```python
from build123d import *

# Parameters (mm, degrees)
MODEL_R             = 3.175
BOSS_EXTRUDE1_DEPTH = 3.048
SKETCH2_R           = 1.4224
BOSS_EXTRUDE2_DEPTH = 3.048
SKETCH3_R           = 1.4224
SKETCH3_R_2         = 0.475
CUT_EXTRUDE1_DEPTH  = 47.828124767


with BuildPart() as part:
    # Model → Boss-Extrude1 (new body)
    with BuildSketch(Plane.XY):
        with BuildLine():
            ThreePointArc((-0.616026415, 14.286925194), (-1.042592722, 15.739677645), (-1.800954663, 17.050149187))
            ThreePointArc((-1.800954663, 17.050149187), (-2.148838289, 17.009806554), (-2.495825317, 16.962366609))
            ThreePointArc((-2.495825317, 16.962366609), (-2.904460903, 15.504468994), (-2.956341002, 13.991274707))
            ThreePointArc((-2.956341002, 13.991274707), (-3.556315124, 13.850932921), (-4.149686627, 13.684875627))
            ThreePointArc((-4.149686627, 13.684875627), (-4.924136412, 14.985904462), (-5.984574038, 16.066608185))
            ThreePointArc((-5.984574038, 16.066608185), (-6.311495456, 15.941017851), (-6.635783413, 15.808776154))
            ThreePointArc((-6.635783413, 15.808776154), (-6.669016568, 14.295057536), (-6.342950641, 12.816500973))
            ThreePointArc((-6.342950641, 12.816500973), (-6.88917389, 12.531360786), (-7.422606766, 12.222954996))
            ThreePointArc((-7.422606766, 12.222954996), (-8.496278501, 13.290511787), (-9.792160616, 14.073543103))
            ThreePointArc((-9.792160616, 14.073543103), (-10.077578151, 13.870596369), (-10.358790833, 13.661862153))
            ThreePointArc((-10.358790833, 13.661862153), (-10.014533394, 12.187435039), (-9.331009364, 10.836419348))
            ThreePointArc((-9.331009364, 10.836419348), (-9.789160524, 10.424397166), (-10.229137224, 9.993021149))
            ThreePointArc((-10.229137224, 9.993021149), (-11.534568165, 10.760027378), (-12.98446973, 11.196185548))
            ThreePointArc((-12.98446973, 11.196185548), (-13.210449547, 10.928634304), (-13.430917328, 10.656523107))
            ThreePointArc((-13.430917328, 10.656523107), (-12.730800257, 9.314031176), (-11.732766451, 8.175445642))
            ThreePointArc((-11.732766451, 8.175445642), (-12.0740582, 7.662430334), (-12.39293337, 7.135189032))
            ThreePointArc((-12.39293337, 7.135189032), (-13.84809849, 7.553450876), (-15.360916858, 7.615330478))
            ThreePointArc((-15.360916858, 7.615330478), (-15.513259815, 7.299985954), (-15.659129891, 6.981595523))
            ThreePointArc((-15.659129891, 6.981595523), (-14.647144119, 5.85539248), (-13.397310672, 5.000778618))
            ThreePointArc((-13.397310672, 5.000778618), (-13.600298394, 4.419004823), (-13.778035935, 3.829026746))
            ThreePointArc((-13.778035935, 3.829026746), (-15.291501858, 3.872263276), (-16.772181085, 3.555976188))
            ThreePointArc((-16.772181085, 3.555976188), (-16.841314914, 3.212652639), (-16.903421733, 2.867988616))
            ThreePointArc((-16.903421733, 2.867988616), (-15.643154047, 2.02883794), (-14.220052592, 1.511894283))
            ThreePointArc((-14.220052592, 1.511894283), (-14.271981822, 0.897916987), (-14.297413829, 0.282272628))
            ThreePointArc((-14.297413829, 0.282272628), (-15.774083925, -0.052232867), (-17.129587491, -0.726813165))
            ThreePointArc((-17.129587491, -0.726813165), (-17.111168259, -1.076543457), (-17.085609422, -1.425824564))
            ThreePointArc((-17.085609422, -1.425824564), (-15.656247076, -1.92519595), (-14.14929631, -2.071987931))
            ThreePointArc((-14.14929631, -2.071987931), (-14.046904143, -2.679590275), (-13.918432631, -3.282217718))
            ThreePointArc((-13.918432631, -3.282217718), (-15.265522286, -3.973447027), (-16.410678917, -4.963934173))
            ThreePointArc((-16.410678917, -4.963934173), (-16.305863972, -5.298096369), (-16.194245434, -5.630047943))
            ThreePointArc((-16.194245434, -5.630047943), (-14.68560052, -5.758262697), (-13.189487703, -5.525679522))
            ThreePointArc((-13.189487703, -5.525679522), (-12.939207816, -6.088729025), (-12.664905121, -6.640474253))
            ThreePointArc((-12.664905121, -6.640474253), (-13.797771739, -7.644994897), (-14.660627033, -8.889152941))
            ThreePointArc((-14.660627033, -8.889152941), (-14.476002283, -9.1867504), (-14.285337446, -9.480514703))
            ThreePointArc((-14.285337446, -9.480514703), (-12.792203675, -9.229516622), (-11.400935076, -8.632172348))
            ThreePointArc((-11.400935076, -8.632172348), (-11.018493474, -9.115290538), (-10.615595045, -9.581485369))
            ThreePointArc((-10.615595045, -9.581485369), (-11.46305645, -10.836179621), (-11.989394033, -12.255833538))
            ThreePointArc((-11.989394033, -12.255833538), (-11.736560131, -12.498167117), (-11.47882917, -12.735285858))
            ThreePointArc((-11.47882917, -12.735285858), (-10.095025626, -12.120846074), (-8.896019768, -11.196274037))
            ThreePointArc((-8.896019768, -11.196274037), (-8.405446665, -11.569104823), (-7.899268091, -11.920456521))
            ThreePointArc((-7.899268091, -11.920456521), (-8.408075165, -13.346487327), (-8.564823313, -14.85243504))
            ThreePointArc((-8.564823313, -14.85243504), (-8.259666742, -15.024278029), (-7.95106384, -15.189852165))
            ThreePointArc((-7.95106384, -15.189852165), (-6.76353999, -14.25057819), (-5.832134822, -13.056872652))
            ThreePointArc((-5.832134822, -13.056872652), (-5.264254728, -13.295989703), (-4.686601071, -13.510421549))
            ThreePointArc((-4.686601071, -13.510421549), (-4.824783595, -15.018186149), (-4.602093245, -16.515803425))
            ThreePointArc((-4.602093245, -16.515803425), (-4.263788115, -16.606358298), (-3.923703928, -16.689984197))
            ThreePointArc((-3.923703928, -16.689984197), (-3.007076261, -15.484894068), (-2.401795395, -14.097059939))
            ThreePointArc((-2.401795395, -14.097059939), (-1.792290307, -14.187438652), (-1.17945767, -14.251477104))
            ThreePointArc((-1.17945767, -14.251477104), (-0.938333127, -15.746237102), (-0.350196733, -17.14142314))
            ThreePointArc((-0.350196733, -17.14142314), (0, -17.145), (0.350196733, -17.14142314))
            ThreePointArc((0.350196733, -17.14142314), (0.938333127, -15.746237102), (1.17945767, -14.251477104))
            ThreePointArc((1.17945767, -14.251477104), (11.018493474, -9.115290538), (14.220052592, 1.511894283))
            ThreePointArc((14.220052592, 1.511894283), (15.643154047, 2.02883794), (16.903421733, 2.867988616))
            ThreePointArc((16.903421733, 2.867988616), (16.841314914, 3.212652639), (16.772181085, 3.555976188))
            ThreePointArc((16.772181085, 3.555976188), (15.291501858, 3.872263276), (13.778035935, 3.829026746))
            ThreePointArc((13.778035935, 3.829026746), (13.600298394, 4.419004823), (13.397310672, 5.000778619))
            ThreePointArc((13.397310672, 5.000778618), (14.647144119, 5.85539248), (15.659129891, 6.981595523))
            ThreePointArc((15.659129891, 6.981595523), (15.513259815, 7.299985954), (15.360916858, 7.615330478))
            ThreePointArc((15.360916858, 7.615330478), (13.84809849, 7.553450876), (12.39293337, 7.135189032))
            ThreePointArc((12.39293337, 7.135189032), (12.0740582, 7.662430334), (11.732766451, 8.175445642))
            ThreePointArc((11.732766451, 8.175445642), (12.730800257, 9.314031176), (13.430917328, 10.656523107))
            ThreePointArc((13.430917328, 10.656523107), (13.210449547, 10.928634304), (12.98446973, 11.196185548))
            ThreePointArc((12.98446973, 11.196185548), (11.534568165, 10.760027378), (10.229137224, 9.993021149))
            ThreePointArc((10.229137224, 9.993021149), (9.789160524, 10.424397166), (9.331009364, 10.836419348))
            ThreePointArc((9.331009364, 10.836419348), (10.014533394, 12.187435039), (10.358790833, 13.661862153))
            ThreePointArc((10.358790833, 13.661862153), (10.077578151, 13.870596369), (9.792160616, 14.073543103))
            ThreePointArc((9.792160616, 14.073543103), (8.496278501, 13.290511787), (7.422606766, 12.222954996))
            ThreePointArc((7.422606766, 12.222954996), (6.88917389, 12.531360786), (6.342950641, 12.816500974))
            ThreePointArc((6.342950641, 12.816500973), (6.669016568, 14.295057536), (6.635783413, 15.808776154))
            ThreePointArc((6.635783413, 15.808776154), (6.311495456, 15.941017851), (5.984574038, 16.066608185))
            ThreePointArc((5.984574038, 16.066608185), (4.924136412, 14.985904462), (4.149686627, 13.684875627))
            ThreePointArc((4.149686627, 13.684875628), (3.556315124, 13.850932921), (2.956341002, 13.991274707))
            ThreePointArc((2.956341002, 13.991274707), (2.904460903, 15.504468994), (2.495825317, 16.962366609))
            ThreePointArc((2.495825317, 16.962366609), (2.148838289, 17.009806554), (1.800954663, 17.050149187))
            ThreePointArc((1.800954663, 17.050149187), (1.042592722, 15.739677645), (0.616026415, 14.286925194))
            ThreePointArc((0.616026415, 14.286925194), (0, 14.3002), (-0.616026415, 14.286925194))
        make_face()
        with Locations(Location((0, 0, 0), (0, 0, 180))):
            Circle(MODEL_R, mode=Mode.SUBTRACT)
    extrude(amount=BOSS_EXTRUDE1_DEPTH)

    # Sketch2 → Boss-Extrude2 (add)
    with BuildSketch(Plane(origin=(0, 0, 0), x_dir=(-1, 0, 0), z_dir=(0, 0, -1))):
        with BuildLine():
            Line((-30.964694704, -25.359415647), (-8.63932874, -11.395513106))
            ThreePointArc((-8.63932874, -11.395513106), (-12.123969987, -7.58320986), (-14.027044449, -2.781680078))
            Line((-14.027044449, -2.781680078), (-36.352410413, -16.745582618))
            ThreePointArc((-36.352410413, -16.745582618), (-37.965469072, -23.746356987), (-30.964694704, -25.359415647))
        make_face()
        with Locations((-33.658552558, -21.052499132)):
            Circle(SKETCH2_R, mode=Mode.SUBTRACT)
    extrude(amount=-BOSS_EXTRUDE2_DEPTH)

    # Sketch3 → Cut-Extrude1 (cut, through all)
    # profile 1 of 6: a face of its own
    with BuildSketch(Plane.XY.offset(3.048)):
        with Locations((-5.710055654, 3.571482805)):
            Circle(SKETCH3_R)
        with Locations((-5.710055654, 3.571482805)):
            Circle(SKETCH3_R_2, mode=Mode.SUBTRACT)
    # profile 2 of 6: a face of its own
    with BuildSketch(Plane.XY.offset(3.048)):
        with Locations((3.557960487, 5.68843629)):
            Circle(SKETCH3_R)
        with Locations((3.557960487, 5.68843629)):
            Circle(SKETCH3_R_2, mode=Mode.SUBTRACT)
    # profile 3 of 6: a face of its own
    with BuildSketch(Plane.XY.offset(3.048)):
        with Locations((-5.710055654, 3.571482805)):
            Circle(SKETCH3_R_2)
    # profile 4 of 6: a face of its own
    with BuildSketch(Plane.XY.offset(3.048)):
        with Locations((3.557960487, 5.68843629)):
            Circle(SKETCH3_R_2)
    # profile 5 of 6: a face of its own
    with BuildSketch(Plane.XY.offset(3.048)):
        with Locations((5.710055654, -3.571482805)):
            Circle(SKETCH3_R)
    # profile 6 of 6: a face of its own
    with BuildSketch(Plane.XY.offset(3.048)):
        with Locations((-3.557960487, -5.68843629)):
            Circle(SKETCH3_R)
    extrude(amount=-CUT_EXTRUDE1_DEPTH, mode=Mode.SUBTRACT)


solid = part.part
```
Check sheet for the modelled part. Datum: model origin and axes. Units: mm. A direction names the side the tool comes from. Coordinates: 2 decimals unless noted, no trailing zeros. Write each loop counter-clockwise with the first axis right and the second up, starting at its lowest first coordinate (ties: lowest second). Pieces come first, ordered by that corner, then holes. Notation, with made-up numbers: M 22,-5 L 67,-5 A15 cw 67,19 Z; hole C 45,-27 d8. An arc over 180 degrees is marked long. Write item = value, one per line. Start each with the question number.
1. Sectioned sample at C-C (x = 26). Record the cut outline in (y, z).
2. Tool access check on faces 1 (the cylindrical face through (-13.784, -7.629, 1.503)), 2 (the cylindrical face through (8.51, 13.3, 1.5)), 3 (the cylindrical face through (2.91, 15.48, 1.5)), 4 (the cylindrical face through (5.06, -13.375, 1.503)), 5 (the cylindrical face through (14.63, 5.84, 1.5)). Record the directions out of +Z, -Z, +X, -X, +Y, -Y that give a thin tool (end or side, any length) a straight path to the whole face; none if there is none.
3. Go/stop test with a flat-tipped pin: pin 1 (2 mm diameter, centred on x = -3.5, y = -9, fed in from -Z). Record where the tip stops, or that it passes through.
4. Thickness scan on probe 1 along X at (y, z) = (15, 0.6); probe 2 along Y at (x, z) = (12, 0.75); probe 3 along Y at (x, z) = (4.5, 2.05). Record the ranges inside material, lowest first.
5. Sectioned sample at B-B (z = 1.85). State how many separate pieces and enclosed holes the cut face has, then the cut area to 3 significant figures.
6. Mould release check, pull along Y, two halves, no side actions. Record for faces 6 (the cylindrical face through (-14.71, -5.76, 1.5)), 7 (the cylindrical face through (0.93, -15.77, 1.5)), 8 (the cylindrical face through (1.05, 15.76, 1.5)): pulls with the +Y half, pulls with the -Y half, needs draft (parallel to the pull), parting line crosses it, or undercut.
7. Sectioned sample at A-A (x = 34.5). Record the cut outline in (y, z).
The answers:
q1.outline = M -22.25,0 L -10.27,0 L -10.27,3.05 L -22.25,3.05 Z
q2.face_1 = +Z, -Z, -X
q2.face_2 = +Z, -Z, +Y
q2.face_3 = +Z, -Z
q2.face_4 = +Z, -Z, -Y
q2.face_5 = +Z, -Z, +X
q3.pin_1 = 0
q4.probe_1 = -6.7 to -4.94, -2.96 to -0.78, 0.78 to 2.96, 4.94 to 6.7
q4.probe_2 = -13.5 to 7.78, 8.43 to 10.94
q4.probe_3 = -13.57 to -4.32, -2.82 to 4.62, 6.75 to 14.36
q5.separate_pieces = 1
q5.enclosed_holes = 6
q5.area = 977 mm²
q6.face_6 = undercut
q6.face_7 = pulls with the -Y half
q6.face_8 = pulls with the +Y half
q7.outline = M -26.06,0 L -22.2,0 L -22.2,3.05 L -26.06,3.05 Z; M -19.91,0 L -15.59,0 L -15.59,3.05 L -19.91,3.05 Z
